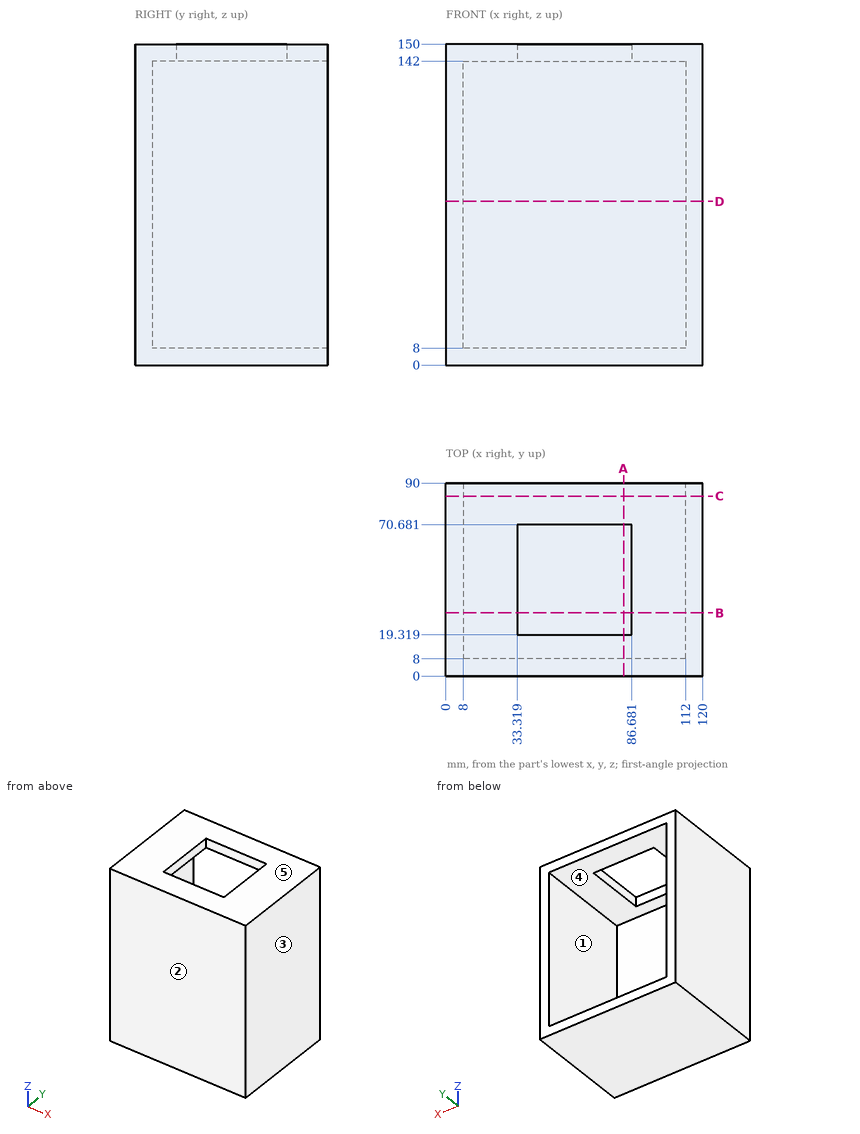
Source: three-view drawing plus pictorial views. Frame: mm from the lowest corner of the part. A direction names the side the tool comes from. Coordinates: 2 decimals unless noted, no trailing zeros. Loops run counter-clockwise (first coordinate to the right, second up) from the corner with the lowest first, then second, coordinate; pieces in that order, holes last. Notation, with made-up numbers: (72, -39.75) -> (111, -39.75) arc R28 cw to (111, -7.75) -> close; hole circle Ø7 at (53, 55). An arc over 180 degrees is marked (long way). Answer in a Markdown table with one row per item. Add a question column.
Q1. Section A-A on x = 83. Return the cut outline in (y, z), and give its area (3 significant figures).
Q2. Section C-C on y = 84. Return the cut outline in (x, z), and give its area (3 significant figures).
Q3. Reachability of the marked faces 1 and 2 from +Z, -Z, +X, -X, +Y, -Y: full face, straight path, thin tool, end or side. Return the list, or none.
Q4. Pull-direction query (X, two-part tool) for the marked faces 3, 4 and 5; classes: pulls with the +X half, pulls with the -X half, needs draft (parallel to the pull), parting line crosses it, or undercut.
Q5. Ray query, line 1 along X through (y, z) = (42, 89.5); line 2 along Y through (x, z) = (74, 144.5); line 3 along Z through (x, y) = (10, 15). Return the intervals inside material, ascending.
Q6. Section B-B on y = 29.5. Return the cut outline in (x, z), and give its area (3 significant figures).
Q7. Contact query for flat-ended pins moving along their axis: pin 1 Ø5 at (x, z) = (59, 129) entering from +Y; pin 2 Ø10 at (x, y) = (73, 15) entering from -Z. Output: stop coordinate, or through.
Q8. Section D-D on z = 76.5. Return the cut outline in (x, y).
Computed values:
| question | item | result |
|---|---|---|
| 1 | outline | (0, 0) -> (90, 0) -> (90, 8) -> (8, 8) -> (8, 142) -> (19.32, 142) -> (19.32, 150) -> (0, 150) -> close; (70.68, 142) -> (90, 142) -> (90, 150) -> (70.68, 150) -> close |
| 1 | area | 2,100 mm^2 |
| 2 | outline | (0, 0) -> (120, 0) -> (120, 150) -> (0, 150) -> close; hole (8, 8) -> (112, 8) -> (112, 142) -> (8, 142) -> close |
| 2 | area | 4,060 mm^2 |
| 3 | face 1 | +Y |
| 3 | face 2 | +Z, -Z, +X, -X, -Y |
| 4 | face 3 | pulls with the +X half |
| 4 | face 4 | undercut |
| 4 | face 5 | needs draft |
| 5 | line 1 | x = 0 to 8, 112 to 120 |
| 5 | line 2 | y = 0 to 19.32, 70.68 to 90 |
| 5 | line 3 | z = 0 to 8, 142 to 150 |
| 6 | outline | (0, 0) -> (120, 0) -> (120, 150) -> (86.68, 150) -> (86.68, 142) -> (112, 142) -> (112, 8) -> (8, 8) -> (8, 142) -> (33.32, 142) -> (33.32, 150) -> (0, 150) -> close |
| 6 | area | 3,640 mm^2 |
| 7 | pin 1 | stops at y = 8 |
| 7 | pin 2 | stops at z = 0 |
| 8 | outline | (0, 0) -> (120, 0) -> (120, 90) -> (112, 90) -> (112, 8) -> (8, 8) -> (8, 90) -> (0, 90) -> close |
